from build123d import *

# Parameters (mm, degrees)
SKETCH1_W            = 140
SKETCH1_H            = 60
BOSS_EXTRUDE2_DEPTH  = 30
SKETCH2_W            = 42
SKETCH2_H            = 23
CUT_EXTRUDE1_DEPTH   = 80
SKETCH3_W            = 60
SKETCH3_H            = 60
BOSS_EXTRUDE3_DEPTH  = 23
CUT_EXTRUDE6_DEPTH   = 156.241746963
SKETCH15_W           = 60
SKETCH15_H           = 30
BOSS_EXTRUDE9_DEPTH  = 20
SKETCH16_W           = 20
SKETCH16_H           = 60
BOSS_EXTRUDE10_DEPTH = 23
CUT_EXTRUDE9_DEPTH   = 162.273060367
CUT_EXTRUDE11_DEPTH  = 162.273060367
SKETCH20_W           = 17.5305996
SKETCH20_H           = 53
BOSS_EXTRUDE11_DEPTH = 60
CUT_EXTRUDE12_DEPTH  = 156.241746963
FILLET8_R            = 8
FILLET9_R            = 8
SKETCH22_W           = 30
SKETCH22_H           = 10
CUT_EXTRUDE13_DEPTH  = 133.454739954
FILLET11_R           = 5
SKETCH23_W           = 8
SKETCH23_H           = 20
CUT_EXTRUDE14_DEPTH  = 35
SKETCH24_W           = 30
SKETCH24_H           = 10
CUT_EXTRUDE15_DEPTH  = 35
FILLET12_R           = 5


with BuildPart() as part:
    # Sketch1 → Boss-Extrude2 (new body)
    with BuildSketch(Plane(origin=(0, 0, 0), x_dir=(1, 0, 0), z_dir=(0, 1, 0))):
        with Locations((70, 30)):
            Rectangle(SKETCH1_W, SKETCH1_H)
    extrude(amount=BOSS_EXTRUDE2_DEPTH)

    # Sketch2 → Cut-Extrude1 (cut)
    with BuildSketch(Plane.ZY):
        with Locations((-30, 11.5)):
            Rectangle(SKETCH2_W, SKETCH2_H)
    extrude(amount=-CUT_EXTRUDE1_DEPTH, mode=Mode.SUBTRACT)

    # Sketch3 → Boss-Extrude3 (add)
    with BuildSketch(Plane.XZ):
        with Locations((110, -30)):
            Rectangle(SKETCH3_W, SKETCH3_H)
    extrude(amount=BOSS_EXTRUDE3_DEPTH)

    # Sketch4 → Cut-Extrude6 (cut, through all)
    with BuildSketch(Plane.XY):
        Polygon((140, -7.341177678), (80, 30), (140, 30), align=None)
    extrude(amount=-CUT_EXTRUDE6_DEPTH, mode=Mode.SUBTRACT)

    # Sketch15 → Boss-Extrude9 (add)
    with BuildSketch(Plane.ZY):
        with Locations((-30, 15)):
            Rectangle(SKETCH15_W, SKETCH15_H)
    extrude(amount=BOSS_EXTRUDE9_DEPTH)

    # Sketch16 → Boss-Extrude10 (add)
    with BuildSketch(Plane.XZ):
        with Locations((-10, -30)):
            Rectangle(SKETCH16_W, SKETCH16_H)
    extrude(amount=BOSS_EXTRUDE10_DEPTH)

    # Sketch17 → Cut-Extrude9 (cut, through all)
    with BuildSketch(Plane.XZ.offset(23)):
        Polygon((80, -60), (140, -50), (140, -60), align=None)
    extrude(amount=-CUT_EXTRUDE9_DEPTH, mode=Mode.SUBTRACT)

    # Sketch18 → Cut-Extrude11 (cut, through all)
    with BuildSketch(Plane.XZ.offset(23)):
        Polygon((80, 0), (140, -10), (140, 0), align=None)
    extrude(amount=-CUT_EXTRUDE11_DEPTH, mode=Mode.SUBTRACT)

    # Sketch20 → Boss-Extrude11 (add, through all)
    with BuildSketch(Plane(origin=(0, 0, -60), x_dir=(-1, 0, 0), z_dir=(0, 0, -1))):
        with Locations((28.7652998, 3.5)):
            Rectangle(SKETCH20_W, SKETCH20_H)
    extrude(amount=-BOSS_EXTRUDE11_DEPTH)

    # Sketch21 → Cut-Extrude12 (cut, through all)
    with BuildSketch(Plane(origin=(0, 0, -60), x_dir=(-1, 0, 0), z_dir=(0, 0, -1))):
        Polygon((18.7652998, -23), (37.5305996, 30), (37.5305996, -23), align=None)
    extrude(amount=-CUT_EXTRUDE12_DEPTH, mode=Mode.SUBTRACT)

    # Fillet8
    # the kernel refuses this fillet: 8 mm, written as the material it takes off along each edge
    with BuildSketch(Plane(origin=(-26.211462289, 22, -52), x_dir=(0, 1, 0), z_dir=(0, 0, -1))) as fillet8_piece_1_section:
        Polygon((0, 0), (FILLET8_R, 0), (FILLET8_R, -FILLET8_R * 1.41489216391), (-FILLET8_R * 0.333759690599, -FILLET8_R * 0.942658193054), align=None)
    fillet8_piece_1 = extrude(amount=FILLET8_R, mode=Mode.PRIVATE)
    fillet8_piece_1 = fillet8_piece_1 - Plane(origin=(-26.211462289, 22, -52), x_dir=(0.816627115211936, -0.5771656215512417, 0), z_dir=(0, 0, -1)) * Sphere(FILLET8_R, mode=Mode.PRIVATE)
    add(fillet8_piece_1, mode=Mode.SUBTRACT)
    with BuildSketch(Plane(origin=(-26.211462289, 22, -8), x_dir=(0, 1, 0), z_dir=(0, 0, 1))) as fillet8_piece_2_section:
        Polygon((0, 0), (FILLET8_R, 0), (FILLET8_R, FILLET8_R * 1.41489216391), (-FILLET8_R * 0.333759690599, FILLET8_R * 0.942658193054), align=None)
    fillet8_piece_2 = extrude(amount=FILLET8_R, mode=Mode.PRIVATE)
    fillet8_piece_2 = fillet8_piece_2 - Plane(origin=(-26.211462289, 22, -8), x_dir=(0.816627115211936, -0.5771656215512417, 0), z_dir=(0, 0, 1)) * Sphere(FILLET8_R, mode=Mode.PRIVATE)
    add(fillet8_piece_2, mode=Mode.SUBTRACT)
    with BuildSketch(Plane(origin=(-37.5305996, 30, -52), x_dir=(1, 0, 0), z_dir=(0, 0, 1))) as fillet8_piece_3:
        with BuildLine():
            CenterArc((FILLET8_R * 1.41489216391, -FILLET8_R), FILLET8_R, 90, 109.497133014)
            Line((FILLET8_R * 0.472233970858, -FILLET8_R * 1.3337596906), (0, 0))
            Line((0, 0), (FILLET8_R * 1.41489216391, 0))
        make_face()
    extrude(amount=44, mode=Mode.SUBTRACT)
    with BuildSketch(Plane(origin=(-33.752727833, 19.329922475, 0), x_dir=(0, 0, -1), z_dir=(0.3337596905987375, -0.9426581930537893, 0))) as fillet8_piece_4:
        with BuildLine():
            CenterArc((FILLET8_R, FILLET8_R), FILLET8_R, 180, 90)
            Line((0, FILLET8_R), (0, 0))
            Line((0, 0), (FILLET8_R, 0))
        make_face()
    extrude(amount=64.904847576, mode=Mode.SUBTRACT)
    with BuildSketch(Plane(origin=(-18.7652998, -23, -74.135352863), x_dir=(-0.33375969059873745, 0.9426581930537893, 0), z_dir=(0, 0, 1))) as fillet8_piece_5:
        with BuildLine():
            CenterArc((FILLET8_R * 0.706767643151, -FILLET8_R), FILLET8_R, 90, 70.502866986)
            Line((-FILLET8_R * 0.235890549903, -FILLET8_R * 0.666240309401), (0, 0))
            Line((0, 0), (FILLET8_R * 0.706767643151, 0))
        make_face()
    extrude(amount=88.270705726, mode=Mode.SUBTRACT)
    with BuildSketch(Plane(origin=(-12.090105988, -41.853163861, -60), x_dir=(0.9426581930537893, 0.3337596905987375, 0), z_dir=(-0.3337596905987375, 0.9426581930537893, 0))) as fillet8_piece_6:
        with BuildLine():
            CenterArc((FILLET8_R, -FILLET8_R), FILLET8_R, 90, 90)
            Line((0, -FILLET8_R), (0, 0))
            Line((0, 0), (FILLET8_R, 0))
        make_face()
    extrude(amount=64.904847576, mode=Mode.SUBTRACT)
    with BuildSketch(Plane(origin=(-26.211462289, 30, -60), x_dir=(0, -1, 0), z_dir=(1, 0, 0)), Plane(origin=(-26.211462289, 30, 0), x_dir=(0, 0, -1), z_dir=(1, 0, 0))) as fillet8_piece_7:
        with BuildLine():
            CenterArc((FILLET8_R, -FILLET8_R), FILLET8_R, 90, 90)
            Line((0, -FILLET8_R), (0, 0))
            Line((0, 0), (FILLET8_R, 0))
        make_face()
    extrude(amount=166.211462289, mode=Mode.SUBTRACT)
    with BuildSketch(Plane(origin=(80, 30, 5.715305101), x_dir=(-1, 0, 0), z_dir=(0, 0, -1))) as fillet8_piece_8:
        with BuildLine():
            CenterArc((FILLET8_R * 0.285765255038, -FILLET8_R), FILLET8_R, 90, 31.896191579)
            Line((-FILLET8_R * 0.24261664781, -FILLET8_R * 0.150993189225), (0, 0))
            Line((0, 0), (FILLET8_R * 0.285765255038, 0))
        make_face()
    extrude(amount=71.430610202, mode=Mode.SUBTRACT)

    # Fillet9
    # the kernel refuses this fillet: 8 mm, written as the material it takes off along each edge
    with BuildSketch(Plane(origin=(132, -11.785128809, -43.222983293), x_dir=(-0.48401910269158954, 0.8713310986405968, -0.08066985044859834), z_dir=(0.7927787698772593, 0.3976147054703528, -0.46195710626163544))) as fillet9_piece_1_section:
        Polygon((-13.665079079, -13.665079079), (13.665079079, -13.665079079), (13.665079079, 13.665079079), (-13.665079079, 13.665079079), align=None)
    fillet9_piece_1 = extrude(amount=13.665079079, mode=Mode.PRIVATE)
    fillet9_piece_1 = split(fillet9_piece_1, bisect_by=Plane(origin=(132, -11.785128809, -43.222983293), z_dir=(0.8406327066696059, -0.5231702543590824, 0.1401054511116011)), keep=Keep.TOP, mode=Mode.PRIVATE)
    fillet9_piece_1 = split(fillet9_piece_1, bisect_by=Plane(origin=(132, -11.785128809, -43.222983293), z_dir=(0, 0, -1)), keep=Keep.TOP, mode=Mode.PRIVATE)
    fillet9_piece_1 = split(fillet9_piece_1, bisect_by=Plane(origin=(132, -11.785128809, -43.222983293), z_dir=(0, 1, 0)), keep=Keep.TOP, mode=Mode.PRIVATE)
    fillet9_piece_1 = split(fillet9_piece_1, bisect_by=Plane(origin=(133.315191898, -11.785128809, -51.114134684), z_dir=(-0.16439898730535743, 0, 0.9863939238321437)), keep=Keep.TOP, mode=Mode.PRIVATE)
    fillet9_piece_1 = split(fillet9_piece_1, bisect_by=Plane(origin=(136.227055223, -4.993074323, -43.222983293), z_dir=(-0.5283819028475878, -0.8490068107754862, 0)), keep=Keep.TOP, mode=Mode.PRIVATE)
    fillet9_piece_1 = split(fillet9_piece_1, bisect_by=Plane(origin=(140, -11.785128809, -43.222983293), z_dir=(-1, 0, 0)), keep=Keep.TOP, mode=Mode.PRIVATE)
    fillet9_piece_1 = fillet9_piece_1 - Plane(origin=(132, -11.785128809, -43.222983293), x_dir=(-0.7927787698772593, -0.3976147054703528, 0.46195710626163544), z_dir=(-0.48401910269158954, 0.8713310986405968, -0.08066985044859834)) * Sphere(FILLET9_R, mode=Mode.PRIVATE)
    add(fillet9_piece_1, mode=Mode.SUBTRACT)
    with BuildSketch(Plane(origin=(132, -11.785128809, -16.777016707), x_dir=(0, 0.7579161794569693, -0.6523519486575872), z_dir=(0.7927787698772593, 0.3976147054703528, 0.46195710626163544))) as fillet9_piece_2_section:
        Polygon((-13.665079079, -13.665079079), (13.665079079, -13.665079079), (13.665079079, 13.665079079), (-13.665079079, 13.665079079), align=None)
    fillet9_piece_2 = extrude(amount=13.665079079, mode=Mode.PRIVATE)
    fillet9_piece_2 = split(fillet9_piece_2, bisect_by=Plane(origin=(132, -11.785128809, -16.777016707), z_dir=(0, 0, 1)), keep=Keep.TOP, mode=Mode.PRIVATE)
    fillet9_piece_2 = split(fillet9_piece_2, bisect_by=Plane(origin=(132, -11.785128809, -16.777016707), z_dir=(0.8406327066696059, -0.5231702543590824, -0.140105451111601)), keep=Keep.TOP, mode=Mode.PRIVATE)
    fillet9_piece_2 = split(fillet9_piece_2, bisect_by=Plane(origin=(132, -11.785128809, -16.777016707), z_dir=(0, 1, 0)), keep=Keep.TOP, mode=Mode.PRIVATE)
    fillet9_piece_2 = split(fillet9_piece_2, bisect_by=Plane(origin=(140, -11.785128809, -16.777016707), z_dir=(-1, 0, 0)), keep=Keep.TOP, mode=Mode.PRIVATE)
    fillet9_piece_2 = split(fillet9_piece_2, bisect_by=Plane(origin=(136.227055223, -4.993074323, -16.777016707), z_dir=(-0.5283819028475878, -0.8490068107754862, 0)), keep=Keep.TOP, mode=Mode.PRIVATE)
    fillet9_piece_2 = split(fillet9_piece_2, bisect_by=Plane(origin=(133.315191898, -11.785128809, -8.885865316), z_dir=(-0.1643989873053573, 0, -0.9863939238321437)), keep=Keep.TOP, mode=Mode.PRIVATE)
    fillet9_piece_2 = fillet9_piece_2 - Plane(origin=(132, -11.785128809, -16.777016707), x_dir=(-0.7927787698772593, -0.3976147054703528, -0.46195710626163544), z_dir=(0, 0.7579161794569693, -0.6523519486575872)) * Sphere(FILLET9_R, mode=Mode.PRIVATE)
    add(fillet9_piece_2, mode=Mode.SUBTRACT)
    with BuildSketch(Plane(origin=(140, -39.942541768, -50), x_dir=(-0.9863939238321437, 0, -0.1643989873053573), z_dir=(0, 1, 0)), Plane(origin=(140, -39.942541768, -10), x_dir=(0, 0, -1), z_dir=(0, 1, 0))) as fillet9_piece_3:
        with BuildLine():
            CenterArc((FILLET9_R * 0.847127088383, FILLET9_R), FILLET9_R, 189.462322208, 80.537677792)
            Line((-FILLET9_R * 0.139266835449, FILLET9_R * 0.835601012695), (0, 0))
            Line((0, 0), (FILLET9_R * 0.847127088383, 0))
        make_face()
    extrude(amount=28.157412959, mode=Mode.SUBTRACT)
    with BuildSketch(Plane(origin=(140, -7.341177678, -16.777016707), x_dir=(0, -1, 0), z_dir=(0, 0, -1))) as fillet9_piece_4:
        with BuildLine():
            CenterArc((FILLET9_R * 0.555493891411, FILLET9_R), FILLET9_R, 211.896191579, 58.103808421)
            Line((-FILLET9_R * 0.293512919364, FILLET9_R * 0.471618097152), (0, 0))
            Line((0, 0), (FILLET9_R * 0.555493891411, 0))
        make_face()
    extrude(amount=26.445966586, mode=Mode.SUBTRACT)
    with BuildSketch(Plane(origin=(137.099294602, -5.535915084, -50.4834509), x_dir=(-0.516051960029516, -0.8522281883121756, -0.08600866000491966), z_dir=(-0.840632706669606, 0.5231702543590825, -0.1401054511116011)), Plane(origin=(137.099294602, -5.535915084, -9.5165491), x_dir=(-0.1189504822205207, 0.07402918485766816, -0.9901365878346354), z_dir=(-0.840632706669606, 0.5231702543590825, 0.140105451111601))) as fillet9_piece_5:
        with BuildLine():
            CenterArc((FILLET9_R * 0.916599247, FILLET9_R), FILLET9_R, 184.983304115, 85.016695885)
            Line((-FILLET9_R * 0.0796208058207, FILLET9_R * 0.913134550261), (0, 0))
            Line((0, 0), (FILLET9_R * 0.916599247, 0))
        make_face()
    extrude(amount=78.609137146, mode=Mode.SUBTRACT)

    # Sketch22 → Cut-Extrude13 (cut, through all)
    with BuildSketch(Plane.ZY.offset(-80)):
        with Locations((-30, -18)):
            Rectangle(SKETCH22_W, SKETCH22_H)
    extrude(amount=-CUT_EXTRUDE13_DEPTH, mode=Mode.SUBTRACT)

    # Fillet11
    fillet11_edges = [part.edges().sort_by_distance(p)[0] for p in [
        (109.900070885, -13, -45),
        (109.900070885, -13, -15),
    ]]
    fillet(fillet11_edges, radius=FILLET11_R)

    # Sketch23 → Cut-Extrude14 (cut)
    with BuildSketch(Plane.XZ.offset(13)):
        with Locations((84, -30)):
            Rectangle(SKETCH23_W, SKETCH23_H)
    extrude(amount=-CUT_EXTRUDE14_DEPTH, mode=Mode.SUBTRACT)

    # Sketch24 → Cut-Extrude15 (cut)
    with BuildSketch(Plane(origin=(0, 0, 0), x_dir=(0, 0, -1), z_dir=(1, 0, 0))):
        with Locations((30, -18)):
            Rectangle(SKETCH24_W, SKETCH24_H)
    extrude(amount=-CUT_EXTRUDE15_DEPTH, mode=Mode.SUBTRACT)

    # Fillet12
    fillet12_edges = [part.edges().sort_by_distance(p)[0] for p in [
        (-11.152961202, -13, -45),
        (-11.152961202, -13, -15),
    ]]
    fillet(fillet12_edges, radius=FILLET12_R)


solid = part.part
Model file for the job. Use its own axes, mm. A direction names the side the tool comes from. Round coordinates to 2 decimals unless told otherwise and drop trailing zeros. Loops run counter-clockwise (first coordinate to the right, second up) from the corner with the lowest first, then second, coordinate; pieces in that order, holes last. Notation, with made-up numbers: (47.25, 31) - (70.25, 31) arc R28 ccw to (70.25, 59) - close; hole circle Ø9 at (82.25, 29.25). An arc over 180 degrees is marked (long way). Write each question's results on one line, items separated by ' | '.
(1) Saw through at A-A, the plane x = -7.5. List the corners of the cut face in (y, z).
Answer below:
outline: (-23, -60) - (22, -60) arc R8 ccw to (30, -52) - (30, -8) arc R8 ccw to (22, 0) - (-23, 0) - (-23, -15) - (-18, -15) arc R5 cw to (-13, -20) - (-13, -40) arc R5 cw to (-18, -45) - (-23, -45) - close
(2) Mould opens along X. For faces 5 (the flat face through (41, 0, -56)), 6 (the cylindrical face through (108.06, 9.99, -6.75)), 7 (the flat face through (26, 30, -30)), 8 (the flat face through (84, 4, -40)) say: released by +X, released by -X, zero draft, split by the parting line, or undercut.
Answer below:
face 5: undercut | face 6: released by +X | face 7: zero draft | face 8: undercut
(3) 3-axis set-ups, long thin cutter, end or side, ignore diameter. For faces 1 (the cylindrical face through (110, -14, -43)), 2 (the flat face through (41, 0, -5)), 3 (the flat face through (84, 4, -20)), 4 (the cylindrical face through (138.053, -17.471, -11.546)): which of +Z, -Z, +X, -X, +Y, -Y reach the whole face in a straight line?
Answer below:
face 1: +X, -X, -Y | face 2: +Z, -Z, -Y | face 3: -Y | face 4: +Z, +X, +Y, -Y
(4) Saw through at B-B, the plane x = 20. List the corners of the cut face in (y, z), then the cut area to 3 significant figures.
Answer below:
outline: (0, -60) - (22, -60) arc R8 ccw to (30, -52) - (30, -8) arc R8 ccw to (22, 0) - (0, 0) - (0, -9) - (23, -9) - (23, -51) - (0, -51) - close | area: 807 mm^2
(5) Wall check: L1, parallel to Z at x = 46.5, y = 10; L2, parallel to Y at x = -7, z = -19.5; L3, parallel to Y at x = 65.5, z = -36. Give the ranges that are in metal, low to high.
Answer below:
L1: z = -60 to -51, -9 to 0 | L2: y = -13.03 to 30 | L3: y = 23 to 30
(6) Pin check, flat tips, straight feed: pin 1 (10 mm diameter, centred on y = 5, z = -33, fed in from -X); pin 2 (10 mm diameter, centred on y = -2.5, z = -20, fed in from -X); pin 3 (22 mm diameter, centred on x = -5.5, z = -26.5, fed in from -Y). Stop position of each tip, or through.
Answer below:
pin 1: stops at x = -30.45 | pin 2: stops at x = -27.79 | pin 3: stops at y = -15.82
